Check sheet for the modelled part. Datum: model origin and axes. Units: mm. A direction names the side the tool comes from. Give positions to 0.01 mm unless a question says otherwise; leave off trailing zeros. Loops run counter-clockwise (first coordinate to the right, second up) from the corner with the lowest first, then second, coordinate; pieces in that order, holes last. Notation, with made-up numbers: (-39.5, 88) -> (-25.5, 88) arc R10 cw to (-25.5, 98) -> close; hole circle Ø6 at (39, -15.75). An arc over 180 degrees is marked (long way). Answer as CSV lines item,"result". Start each with the question number.
(1) Section check A-A on x = -7.25. Enter the section's corners in (y, z).
(2) Material ranges on line 1 (Z direction, x = -8.5, y = 15); line 2 (Z direction, x = -0.25, y = 13); line 3 (Y direction, x = 11.5, z = -0.75), recorded low to high. Write a range as from..to.
(3) Section check C-C on y = 14. Enter the section's corners in (x, z), plus the area to 3 significant figures.
(4) Section check B-B on z = 3.25. Enter the section's corners in (x, y).
(5) Release check for a two-part mould opening along X. For faces 4 (the face through (-11.2, 16.83, 3.01)), 5 (the face through (1.211, 9.86, -7.908)), 6 (the face through (-10, 10, -2)) record: pulls with the +X half, pulls with the -X half, needs draft (parallel to the pull), parting line crosses it, or undercut.
(6) Section check D-D on z = 0. Enter the section's corners in (x, y), plus the area to 3 significant figures.
(7) Gauge pin test, flat ends, axial feed: pin 1 Ø6.5 at (x, y) = (-10.93, 5.2) entering from -Z; pin 2 Ø9.5 at (x, z) = (0, 0) entering from -Y; pin 3 Ø4.5 at (x, y) = (-8, 14.5) entering from -Z; pin 4 Ø5.5 at (x, y) = (11.17, 14) entering from +Z. Record the tip position at first contact, or that the pin passes through.
(8) Access from +Z, -Z, +X, -X, +Y, -Y to the whole of each face (thin tool, end or side, straight path). Record for faces 1 (the face through (11, 10, 2)), 2 (the face through (-11, 10, -4)), 3 (the face through (-11, 10, 4)).
from build123d import *

# Parameters (mm, degrees)
BOSS_EXTRUDE1_DEPTH = 20
SKETCH2_R           = 2.05
CUT_EXTRUDE1_DEPTH  = 20


with BuildPart() as part:
    # Sketch1 → Boss-Extrude1 (new body)
    with BuildSketch(Plane(origin=(0, 0, 0), x_dir=(1, 0, 0), z_dir=(0, 1, 0))):
        with BuildLine():
            Line((-14.92820323, 2), (-5.656854249, 2))
            ThreePointArc((-5.656854249, 2), (6, 0), (-5.656854249, -2))
            Line((-5.656854249, -2), (-14.92820323, -2))
            Line((-14.92820323, -2), (-14.92820323, -4))
            Line((-14.92820323, -4), (-6.92820323, -4))
            ThreePointArc((-6.92820323, -4), (1.080363027, -7.926715318), (7.745966692, -2))
            Line((7.745966692, -2), (14.745966692, -2))
            Line((14.745966692, -2), (14.745966692, 2))
            Line((14.745966692, 2), (7.745966692, 2))
            ThreePointArc((7.745966692, 2), (1.080363027, 7.926715318), (-6.92820323, 4))
            Line((-6.92820323, 4), (-14.92820323, 4))
            Line((-14.92820323, 4), (-14.92820323, 2))
        make_face()
    extrude(amount=BOSS_EXTRUDE1_DEPTH)

    # Sketch2 → Cut-Extrude1 (cut)
    with BuildSketch(Plane.XY.offset(4)):
        with Locations((-10.92820323, 14.8)):
            Circle(SKETCH2_R)
        with Locations((-10.92820323, 5.2)):
            Circle(SKETCH2_R)
        with Locations((11.170658207, 14)):
            Circle(SKETCH2_R)
        with Locations((11.170658207, 6)):
            Circle(SKETCH2_R)
    extrude(amount=-CUT_EXTRUDE1_DEPTH, mode=Mode.SUBTRACT)


solid = part.part
Working result:
1,outline,"(0, -4) -> (20, -4) -> (20, -2) -> (0, -2) -> close; (0, 2) -> (20, 2) -> (20, 4) -> (0, 4) -> close"
2,line 1,"z = -4..-2, 2..4"
2,line 2,"z = -8..-5.99, 5.99..8"
2,line 3,"y = 0..3.98, 8.02..11.98, 16.02..20"
3,outline,"(-14.93, -4) -> (-12.82, -4) -> (-12.82, -2) -> (-14.93, -2) -> close; (-14.93, 2) -> (-12.82, 2) -> (-12.82, 4) -> (-14.93, 4) -> close; (-9.04, -4) -> (-6.93, -4) arc R8 ccw to (7.75, -2) -> (9.12, -2) -> (9.12, 2) -> (7.75, 2) arc R8 ccw to (-6.93, 4) -> (-9.04, 4) -> (-9.04, 2) -> (-5.66, 2) arc R6 cw (long way) to (-5.66, -2) -> (-9.04, -2) -> close; (13.22, -2) -> (14.75, -2) -> (14.75, 2) -> (13.22, 2) -> close"
3,area,"106 mm^2"
4,outline,"(-14.93, 0) -> (-5.04, 0) -> (-5.04, 20) -> (-14.93, 20) -> close; (5.04, 0) -> (7.31, 0) -> (7.31, 20) -> (5.04, 20) -> close; hole circle Ø4.1 at (-10.93, 5.2); hole circle Ø4.1 at (-10.93, 14.8)"
5,face 4,"undercut"
5,face 5,"parting line crosses it"
5,face 6,"needs draft"
6,outline,"(6, 0) -> (14.75, 0) -> (14.75, 20) -> (6, 20) -> close; hole circle Ø4.1 at (11.17, 6); hole circle Ø4.1 at (11.17, 14)"
6,area,"149 mm^2"
7,pin 1,"stops at z = -4"
7,pin 2,"passes through"
7,pin 3,"stops at z = -5.56"
7,pin 4,"stops at z = 2"
8,face 1,"+Z, +X, +Y, -Y"
8,face 2,"-Z, -X, +Y, -Y"
8,face 3,"+Z, -X, +Y, -Y"
